Autodesk Inventor part; units mm, degrees
ref_plane "body_screw_XY" through (0, -10, 5) normal (0, 0, 1) x (1, 0, 0)
ref_plane "body_screw_YZ" through (0, -10, 5) normal (1, 0, 0) x (0, 1, 0)
ref_plane "body_screw_ZX" through (0, -10, 5) normal (0, 1, 0) x (0, 0, 1)
sketch "Sketch_1" plane through (0, 0, 0) normal (0, 0, 1) x (1, 0, 0)
  line L0 (5, 0) -> (-5, 0)
  line L1 (-5, 14.5) -> (-5, 6.5)
  line L2 (-5, 6.5) -> (-4.5, 6)
  line L3 (-4.5, 6) -> (4.5, 6)
  line L4 (4.5, 6) -> (5, 6.5)
  line L5 (5, 6.5) -> (5, 14.5)
  line L6 (5, 14.5) -> (4.5, 15)
  line L7 (4.5, 15) -> (-4.5, 15)
  line L8 (-4.5, 15) -> (-5, 14.5)
revolve "Revolution1" add sketch "Sketch_1" angle 360 about axis through (5, 0, 0) along (1, 0, 0)
sketch "Sketch_2" plane through (0, 0, 0) normal (1, 0, 0) x (0, 1, 0)
  line L0 (-15, 0.75) -> (-15, -0.75)
  line L1 (-15, -0.75) -> (9.5, -0.75)
  line L2 (9.5, -0.75) -> (9.5, 0.75)
  line L3 (9.5, 0.75) -> (-15, 0.75)
extrude "Extrusion1" cut sketch "Sketch_2" along normal mid plane 10
sketch "Sketch_3" plane through (0, 0, 0) normal (1, 0, 0) x (0, 1, 0)
  line L0 (-10, 15) -> (-10, 0)
  line L1 (-10, 0) -> (-12.25, 0)
  line L2 (-12.25, 0) -> (-12.25, 5)
  line L3 (-12.25, 5) -> (-13.75, 5)
  line L4 (-13.75, 5) -> (-13.75, 15)
  line L5 (-13.75, 15) -> (-10, 15)
  line L6 (-10, 15) -> (-10, 0)
revolve "Revolution2" cut sketch "Sketch_3" angle 360 about axis through (0, -10, 15) along (0, 0, 1)
sketch "Sketch_4" plane through (0, 0, 0) normal (1, 0, 0) x (0, 1, 0)
  line L0 (-10, -15.75) -> (-10, -0.75)
  line L1 (-10, -0.75) -> (-8, -0.75)
  line L2 (-8, -0.75) -> (-8.379, -1.129)
  line L3 (-8.379, -1.129) -> (-8.379, -15.75)
  line L4 (-8.379, -15.75) -> (-10, -15.75)
  line L5 (-10, -15.75) -> (-10, -0.75)
revolve "Revolution3" cut sketch "Sketch_4" angle 360 about axis through (0, -10, -15.75) along (0, 0, -1)
thread "Thread1"
sketch "Sketch_7" plane through (0, 0, -11) normal (0, 0, 1) x (1, 0, 0)
  line L0 (5, 0) -> (-5, 0)
  line L1 (-5, 0) -> (-5, 2.5)
  line L2 (-5, 2.5) -> (-4.567, 2.067)
  line L3 (-4.567, 2.067) -> (4.567, 2.067)
  line L4 (4.567, 2.067) -> (5, 2.5)
  line L5 (5, 2.5) -> (5, 0)
  line L6 (5, 0) -> (-5, 0)
revolve "Revolution4" cut sketch "Sketch_7" angle 360 about axis through (5, 0, -11) along (1, 0, 0)
thread "Thread2"
sketch "Sketch_8" plane through (0, 0, 11) normal (0, 0, 1) x (1, 0, 0)
  line L0 (5, 0) -> (-5, 0)
  line L1 (-5, 0) -> (-5, 2.5)
  line L2 (-5, 2.5) -> (-4.567, 2.067)
  line L3 (-4.567, 2.067) -> (4.567, 2.067)
  line L4 (4.567, 2.067) -> (5, 2.5)
  line L5 (5, 2.5) -> (5, 0)
  line L6 (5, 0) -> (-5, 0)
revolve "Revolution5" cut sketch "Sketch_8" angle 360 about axis through (5, 0, 11) along (1, 0, 0)
thread "Thread3"
ref_plane "body_screw_XY" through (0, -10, 5) normal (0, 0, 1) x (1, 0, 0)
ref_plane "body_screw_YZ" through (0, -10, 5) normal (1, 0, 0) x (0, 1, 0)
ref_plane "body_screw_ZX" through (0, -10, 5) normal (0, 1, 0) x (0, 0, 1)
properties part number "SCSW12-10b"
Build history of the part. All positions in model axes, mm. A direction names the side the tool comes from. Round coordinates to 2 decimals unless told otherwise and drop trailing zeros. Answer as CSV lines item,"result".
Q1. Tool access for faces 1 (the cylindrical face through (0.487, -8.454, -6.864)), 2 (the conical face through (-4.64, -0.13, 6.14)), 3 (the conical face through (4.64, -0.13, -6.14)), 4 (the cylindrical face through (0, 0, 6)), 5 (the flat face through (0, 8, 0.75)): list every direction of +Z, -Z, +X, -X, +Y, -Y with a clear straight run to the whole face (end or side of a thin tool).
Report:
face 1,"+Z, -Z"
face 2,"-X"
face 3,"+X"
face 4,"+X, -X"
face 5,"+X, -X, -Y"
Q2. Cut at A-A (y = 0). State how many separate pieces and enclosed holes the cut face has, and give its area (3 significant figures).
Report:
separate pieces,"4"
enclosed holes,"0"
area,"95.6 mm^2"
Q3. Drop flat-ended pins along their axis: pin 1 (6 mm diameter, centred on x = 1.5, y = -9, fed in from +Z); pin 2 (5 mm diameter, centred on x = 0, y = -10, fed in from +Z); pin 3 (1.2 mm diameter, centred on x = -1.5, z = 0, fed in from -Y); pin 4 (3.5 mm diameter, centred on y = 0, z = 11, fed in from +X) (3 decimals). Give the stop position or say it passes through.
Report:
pin 1,"stops at z = 13.75"
pin 2,"stops at z = 5"
pin 3,"stops at y = 9.5"
pin 4,"passes through"
Q4. Drill centre lines: probe 1 along Z at (x, y) = (0.25, 0); probe 2 along X at (y, z) = (-10, 8); probe 3 along Y at (x, z) = (-1, 0). Where is each one in solid material? Low to high. Write a range as [from, to].
Report:
probe 1,"z = [-15, -13.07], [-8.93, -6], [6, 8.93], [13.07, 15]"
probe 2,"x = [-5, -3.75], [3.75, 5]"
probe 3,"y = [9.5, 15]"
Q5. Pull direction Y, two halves, no side cores. Call faces 6 (the flat face through (-2, -12, 5)), 7 (the flat face through (0, 9.5, 0)), 8 (the flat face through (0, 8, -0.75)): +Y half, -Y half, draft (parallel to the pull), parting line (faces both ways), or undercut.
Report:
face 6,"undercut"
face 7,"-Y half"
face 8,"draft"
